Read the model definition and answer for the solid it produces. Units are mm, in the model's axes. Face numbers are marked on the shaded views. Coordinates: 2 decimals unless noted, no trailing zeros. Write each loop counter-clockwise with the first axis right and the second up, starting at its lowest first coordinate (ties: lowest second). Pieces come first, ordered by that corner, then holes. Notation, with made-up numbers: (27.5, 61) -> (82.5, 61) arc R14 cw to (82.5, 73) -> close; hole circle Ø4 at (10.25, 31). An arc over 180 degrees is marked (long way). Answer in a Markdown table with one row per item. Add a question column.
Item 1: For a pull along X with two mould halves and no side action, classify the marked faces 1 and 2 as +X half, -X half, draft (parallel to the pull), parting line (faces both ways), or undercut.
Item 2: Section D-D on x = 50 is taken. Write down the section's boundary in (y, z), then the cut area to 3 significant figures.
Item 3: Section A-A on x = 70 is taken. Count the separate pieces of the cut face and the enclosed holes in it, then the cut area to 3 significant figures.
Item 4: Section B-B on x = 6 is taken. Write down the section's boundary in (y, z), then the cut area to 3 significant figures.
Item 5: Section C-C on y = 6 is taken. Write down the section's boundary in (x, z), then the cut area to 3 significant figures.
Item 6: Given pin 1 Ø2 at (x, z) = (89.5, 8) entering from -Y; pin 2 Ø6.5 at (x, z) = (77.5, 6) entering from +Y; pin 3 Ø12 at (x, y) = (89, 65.5) entering from +Z; pin 4 Ø6 at (x, y) = (90, 50) entering from -Z, each flat-ended and moving along its own axis, determine where each tip first touches the part or whether it passes through.
Item 7: Straight lines are drawn through the part: line 1 (X direction, y = 94, z = 10.9); line 2 (Y direction, x = 6, z = 10.7); line 3 (X direction, y = 50, z = 1.9). For each, find the intervals that lie inside material, in ascending order. Write a range as from..to.
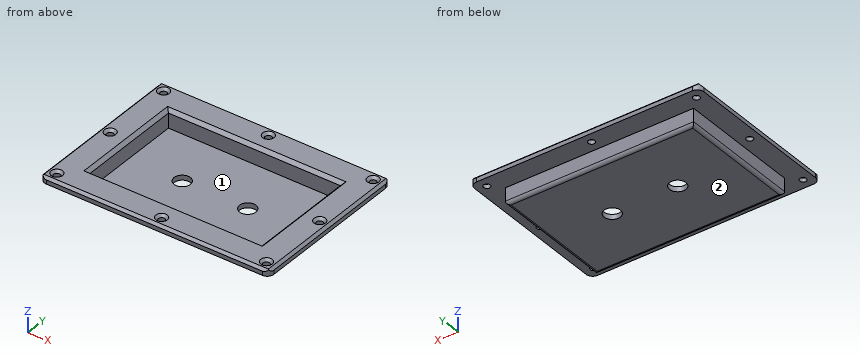
```python
from build123d import *

# Parameters (mm, degrees)
CYLINDER009_R     = 5
CYLINDER009_DEPTH = 20
CYLINDER008_R     = 2
CYLINDER008_DEPTH = 20
CYLINDER007_R     = 2
CYLINDER007_DEPTH = 20
CYLINDER006_R     = 5
CYLINDER006_DEPTH = 20
BOX002_W          = 105
BOX002_H          = 65
BOX002_DEPTH      = 20
BOX001_W          = 115
BOX001_H          = 75
BOX001_DEPTH      = 10
FILLET_R          = 2
CYLINDER003_R     = 2
CYLINDER003_DEPTH = 10
CYLINDER002_R     = 2
CYLINDER002_DEPTH = 10
CYLINDER004_R     = 2
CYLINDER004_DEPTH = 10
CYLINDER005_R     = 2
CYLINDER005_DEPTH = 10
CYLINDER001_R     = 2
CYLINDER001_DEPTH = 10
CYLINDER_R        = 2
CYLINDER_DEPTH    = 10
BOX_W             = 140
BOX_H             = 100
BOX_DEPTH         = 4
CHAMFER_SIZE      = 1.5
CHAMFER001_SIZE   = 2
FILLET001_R       = 4
FILLET002_R       = 4
CHAMFER002_SIZE   = 1.5


with BuildPart() as cylinder009:
    # Cylinder009 → Cylinder009 (new body)
    with BuildSketch(Plane(origin=(90, 50, -5), x_dir=(1, 0, 0), z_dir=(0, 0, 1))):
        Circle(CYLINDER009_R)
    extrude(amount=CYLINDER009_DEPTH)


with BuildPart() as cylinder008:
    # Cylinder008 → Cylinder008 (new body)
    with BuildSketch(Plane(origin=(70, 6, 0), x_dir=(1, 0, 0), z_dir=(0, 0, 1))):
        Circle(CYLINDER008_R)
    extrude(amount=CYLINDER008_DEPTH)


with BuildPart() as cylinder007:
    # Cylinder007 → Cylinder007 (new body)
    with BuildSketch(Plane(origin=(70, 94, 0), x_dir=(1, 0, 0), z_dir=(0, 0, 1))):
        Circle(CYLINDER007_R)
    extrude(amount=CYLINDER007_DEPTH)


with BuildPart() as cylinder006:
    # Cylinder006 → Cylinder006 (new body)
    with BuildSketch(Plane(origin=(50, 50, -5), x_dir=(1, 0, 0), z_dir=(0, 0, 1))):
        Circle(CYLINDER006_R)
    extrude(amount=CYLINDER006_DEPTH)


with BuildPart() as cube002:
    # Box002 → Box002 (new body)
    with BuildSketch(Plane(origin=(17.5, 17.5, 3), x_dir=(1, 0, 0), z_dir=(0, 0, 1))):
        with Locations((52.5, 32.5)):
            Rectangle(BOX002_W, BOX002_H)
    extrude(amount=BOX002_DEPTH)


with BuildPart() as fillet_body:
    # Box001 → Box001 (new body)
    with BuildSketch(Plane(origin=(12.5, 12.5, 0), x_dir=(1, 0, 0), z_dir=(0, 0, 1))):
        with Locations((57.5, 37.5)):
            Rectangle(BOX001_W, BOX001_H)
    extrude(amount=BOX001_DEPTH)

    # Fillet
    fillet_edges = [fillet_body.edges().sort_by_distance(p)[0] for p in [
        (12.5, 50, 0),
        (127.5, 50, 0),
        (70, 12.5, 0),
        (70, 87.5, 0),
    ]]
    fillet(fillet_edges, radius=FILLET_R)


with BuildPart() as cylinder003:
    # Cylinder003 → Cylinder003 (new body)
    with BuildSketch(Plane(origin=(6, 94, 0), x_dir=(1, 0, 0), z_dir=(0, 0, 1))):
        Circle(CYLINDER003_R)
    extrude(amount=CYLINDER003_DEPTH)


with BuildPart() as cylinder002:
    # Cylinder002 → Cylinder002 (new body)
    with BuildSketch(Plane(origin=(6, 50, 0), x_dir=(1, 0, 0), z_dir=(0, 0, 1))):
        Circle(CYLINDER002_R)
    extrude(amount=CYLINDER002_DEPTH)


with BuildPart() as cylinder004:
    # Cylinder004 → Cylinder004 (new body)
    with BuildSketch(Plane(origin=(6, 6, 0), x_dir=(1, 0, 0), z_dir=(0, 0, 1))):
        Circle(CYLINDER004_R)
    extrude(amount=CYLINDER004_DEPTH)


with BuildPart() as cylinder005:
    # Cylinder005 → Cylinder005 (new body)
    with BuildSketch(Plane(origin=(134, 94, 0), x_dir=(1, 0, 0), z_dir=(0, 0, 1))):
        Circle(CYLINDER005_R)
    extrude(amount=CYLINDER005_DEPTH)


with BuildPart() as cylinder001:
    # Cylinder001 → Cylinder001 (new body)
    with BuildSketch(Plane(origin=(134, 50, 0), x_dir=(1, 0, 0), z_dir=(0, 0, 1))):
        Circle(CYLINDER001_R)
    extrude(amount=CYLINDER001_DEPTH)


with BuildPart() as cylinder:
    # Cylinder → Cylinder (new body)
    with BuildSketch(Plane(origin=(134, 6, 0), x_dir=(1, 0, 0), z_dir=(0, 0, 1))):
        Circle(CYLINDER_R)
    extrude(amount=CYLINDER_DEPTH)


with BuildPart() as cut010:
    # Box → Box (new body)
    with BuildSketch(Plane.XY):
        with Locations((70, 50)):
            Rectangle(BOX_W, BOX_H)
    extrude(amount=BOX_DEPTH)

    # Cut: cut Cylinder
    add(cylinder.part, mode=Mode.SUBTRACT)

    # Cut001: cut Cylinder001
    add(cylinder001.part, mode=Mode.SUBTRACT)

    # Cut002: cut Cylinder005
    add(cylinder005.part, mode=Mode.SUBTRACT)

    # Cut003: cut Cylinder004
    add(cylinder004.part, mode=Mode.SUBTRACT)

    # Cut004: cut Cylinder002
    add(cylinder002.part, mode=Mode.SUBTRACT)

    # Cut005: cut Cylinder003
    add(cylinder003.part, mode=Mode.SUBTRACT)


with BuildPart() as cut010_1:
    # Cut005 placement: moved
    add(cut010.part.moved(Location((0, 0, 10))))

    # Chamfer
    chamfer_edges = [cut010_1.edges().sort_by_distance(p)[0] for p in [
        (4, 50, 14),
        (4, 6, 14),
        (0, 50, 14),
        (70, 100, 14),
        (70, 0, 14),
        (140, 50, 14),
        (4, 94, 14),
        (132, 94, 14),
        (132, 50, 14),
        (132, 6, 14),
    ]]
    chamfer(chamfer_edges, length=CHAMFER_SIZE)

    # Fusion: union Fillet body
    add(fillet_body.part)

    # Cut006: cut Cube002
    add(cube002.part, mode=Mode.SUBTRACT)

    # Cut007: cut Cylinder006
    add(cylinder006.part, mode=Mode.SUBTRACT)

    # Chamfer001
    chamfer001_edges = [cut010_1.edges().sort_by_distance(p)[0] for p in [
        (122.5, 50, 14),
        (70, 17.5, 14),
        (17.5, 50, 14),
        (70, 82.5, 14),
    ]]
    chamfer(chamfer001_edges, length=CHAMFER001_SIZE)

    # Fillet001
    fillet001_edges = [cut010_1.edges().sort_by_distance(p)[0] for p in [
        (140, 0, 11.25),
        (140, 100, 11.25),
    ]]
    fillet(fillet001_edges, radius=FILLET001_R)

    # Fillet002
    fillet002_edges = [cut010_1.edges().sort_by_distance(p)[0] for p in [
        (0, 0, 11.25),
        (0, 100, 11.25),
    ]]
    fillet(fillet002_edges, radius=FILLET002_R)

    # Cut008: cut Cylinder007
    add(cylinder007.part, mode=Mode.SUBTRACT)

    # Cut009: cut Cylinder008
    add(cylinder008.part, mode=Mode.SUBTRACT)

    # Chamfer002
    chamfer002_edges = [cut010_1.edges().sort_by_distance(p)[0] for p in [
        (68, 6, 14),
        (68, 94, 14),
    ]]
    chamfer(chamfer002_edges, length=CHAMFER002_SIZE)

    # Cut010: cut Cylinder009
    add(cylinder009.part, mode=Mode.SUBTRACT)


solid = cut010_1.part
```
Results below:
| question | item | result |
|---|---|---|
| 1 | face 1 | undercut |
| 1 | face 2 | draft |
| 2 | outline | (0, 10) -> (12.5, 10) -> (12.5, 2) arc R2 ccw to (14.5, 0) -> (45, 0) -> (45, 3) -> (17.5, 3) -> (17.5, 12) -> (15.5, 14) -> (1.5, 14) -> (0, 12.5) -> close; (55, 0) -> (85.5, 0) arc R2 ccw to (87.5, 2) -> (87.5, 10) -> (100, 10) -> (100, 12.5) -> (98.5, 14) -> (84.5, 14) -> (82.5, 12) -> (82.5, 3) -> (55, 3) -> close |
| 2 | area | 397 mm2 |
| 3 | separate pieces | 3 |
| 3 | enclosed holes | 0 |
| 3 | area | 391 mm2 |
| 4 | outline | (0, 10) -> (4, 10) -> (4, 12.5) -> (2.5, 14) -> (1.5, 14) -> (0, 12.5) -> close; (8, 10) -> (48, 10) -> (48, 12.5) -> (46.5, 14) -> (9.5, 14) -> (8, 12.5) -> close; (52, 10) -> (92, 10) -> (92, 12.5) -> (90.5, 14) -> (53.5, 14) -> (52, 12.5) -> close; (96, 10) -> (100, 10) -> (100, 12.5) -> (98.5, 14) -> (97.5, 14) -> (96, 12.5) -> close |
| 4 | area | 343 mm2 |
| 5 | outline | (0, 10) -> (4, 10) -> (4, 12.5) -> (2.5, 14) -> (1.5, 14) -> (0, 12.5) -> close; (8, 10) -> (68, 10) -> (68, 12.5) -> (66.5, 14) -> (9.5, 14) -> (8, 12.5) -> close; (72, 10) -> (132, 10) -> (132, 12.5) -> (130.5, 14) -> (73.5, 14) -> (72, 12.5) -> close; (136, 10) -> (140, 10) -> (140, 12.5) -> (138.5, 14) -> (137.5, 14) -> (136, 12.5) -> close |
| 5 | area | 503 mm2 |
| 6 | pin 1 | stops at y = 12.5 |
| 6 | pin 2 | stops at y = 87.5 |
| 6 | pin 3 | stops at z = 3 |
| 6 | pin 4 | passes through |
| 7 | line 1 | x = 0..4, 8..68, 72..132, 136..140 |
| 7 | line 2 | y = 0..4, 8..48, 52..92, 96..100 |
| 7 | line 3 | x = 12.5..45, 55..85, 95..127.5 |
